```python
from build123d import *

# Parameters (mm, degrees)
F1_DEPTH   = 2
F2_DEPTH   = 7
F3_SIZE2   = 1.74999
F3_SIZE    = 0.99999
F3_2_SIZE2 = 1.74999
F3_2_SIZE  = 0.99999
F3_3_SIZE2 = 1.74999
F3_3_SIZE  = 0.99999
F3_4_SIZE2 = 1.74999
F3_4_SIZE  = 0.99999


# Not quite as in the source:
# - a fillet or chamfer is up to 0.001 mm smaller than in the source, because OpenCascade refuses the exact size


with BuildPart() as f1:
    # F0 (on Top) → F1 (new body)
    with BuildSketch(Plane.XY):
        with BuildLine():
            ThreePointArc((2.5497759502, -1.5807095255), (2.8852493697, -0.8217883394), (3, 0))
            ThreePointArc((3, 0), (2.6235481729, 1.4549896853), (1.5886700104, 2.544823687))
            ThreePointArc((1.5886700104, 2.544823687), (0.8262956308, 2.8839617769), (0, 3))
            ThreePointArc((0, 3), (-1.6310845521, 2.51784892), (-2.7378829853, 1.226375456))
            ThreePointArc((-2.7378829853, 1.226375456), (-2.9337389928, 0.6270370979), (-3, 0))
            ThreePointArc((-3, 0), (-2.488818496, -1.6750470125), (-1.1294783373, -2.7792586575))
            ThreePointArc((-1.1294783373, -2.7792586575), (-0.5754233343, -2.944297537), (0, -3))
            ThreePointArc((0, -3), (1.4590872872, -2.6212715022), (2.5497759502, -1.5807095255))
        make_face()
        with BuildLine():
            Line((0, -4.75), (0, -3))
            ThreePointArc((0, -3), (-0.5754233343, -2.944297537), (-1.1294783373, -2.7792586575))
            Line((-1.1294783373, -2.7792586575), (-2.0097266443, -4.3038934484))
            ThreePointArc((-2.0097266443, -4.3038934484), (-1.0293216504, -4.6371324048), (0, -4.75))
        make_face()
        with BuildLine():
            Line((4.75, 0), (3, 0))
            ThreePointArc((3, 0), (2.8852493697, -0.8217883394), (2.5497759502, -1.5807095255))
            Line((2.5497759502, -1.5807095255), (4.0657909798, -2.455981211))
            ThreePointArc((4.0657909798, -2.455981211), (4.5757516953, -1.2747534754), (4.75, 0))
        make_face()
        with BuildLine():
            ThreePointArc((-3, 0), (-2.9337389928, 0.6270370979), (-2.7378829853, 1.226375456))
            Line((-2.7378829853, 1.226375456), (-4.2584618162, 2.1042820533))
            ThreePointArc((-4.2584618162, 2.1042820533), (-4.625483414, 1.0804643384), (-4.75, 0))
            Line((-4.75, 0), (-3, 0))
        make_face()
        with BuildLine():
            ThreePointArc((0, 3), (0.8262956308, 2.8839617769), (1.5886700104, 2.544823687))
            Line((1.5886700104, 2.544823687), (2.4639985646, 4.0609372162))
            ThreePointArc((2.4639985646, 4.0609372162), (1.2792670212, 4.5744918722), (0, 4.75))
            Line((0, 4.75), (0, 3))
        make_face()
    extrude(amount=F1_DEPTH)

    # F0 (on Top) → F2 (join)
    with BuildSketch(Plane.XY):
        with BuildLine():
            Line((-2.0097266443, -4.3038934484), (-1.1294783373, -2.7792586575))
            ThreePointArc((-1.1294783373, -2.7792586575), (-2.488818496, -1.6750470125), (-3, 0))
            Line((-3, 0), (-4.75, 0))
            ThreePointArc((-4.75, 0), (-4.0067880877, -2.5511074497), (-2.0097266443, -4.3038934484))
        make_face()
        with BuildLine():
            Line((4.0657909798, -2.455981211), (2.5497759502, -1.5807095255))
            ThreePointArc((2.5497759502, -1.5807095255), (1.4590872872, -2.6212715022), (0, -3))
            Line((0, -3), (0, -4.75))
            ThreePointArc((0, -4.75), (2.334158226, -4.1369318795), (4.0657909798, -2.455981211))
        make_face()
        with BuildLine():
            ThreePointArc((1.5886700104, 2.544823687), (2.6235481729, 1.4549896853), (3, 0))
            Line((3, 0), (4.75, 0))
            ThreePointArc((4.75, 0), (4.1392326089, 2.3300758376), (2.4639985646, 4.0609372162))
            Line((2.4639985646, 4.0609372162), (1.5886700104, 2.544823687))
        make_face()
        with BuildLine():
            ThreePointArc((-2.7378829853, 1.226375456), (-1.6310845521, 2.51784892), (0, 3))
            Line((0, 3), (0, 4.75))
            ThreePointArc((0, 4.75), (-2.5067070278, 4.0347143488), (-4.2584618162, 2.1042820533))
            Line((-4.2584618162, 2.1042820533), (-2.7378829853, 1.226375456))
        make_face()
    extrude(amount=F2_DEPTH)

    # F3 (size 1 and 1.75 in the source; OpenCascade refuses exactly that, so slightly less here)
    f3_edges = [f1.edges().sort_by_distance(p)[0] for p in [
        (-2.488818, -1.675047, 7),
    ]]
    f3_side = f1.faces().sort_by_distance((-2.488818, -1.675047, 4.5))[0]
    chamfer(f3_edges, length=F3_SIZE, length2=F3_SIZE2, reference=f3_side)

    # F3#2 (size 1 and 1.75 in the source; OpenCascade refuses exactly that, so slightly less here)
    f3_2_edges = [f1.edges().sort_by_distance(p)[0] for p in [
        (-1.631085, 2.517849, 7),
    ]]
    f3_2_side = f1.faces().sort_by_distance((-1.631085, 2.517849, 4.5))[0]
    chamfer(f3_2_edges, length=F3_2_SIZE, length2=F3_2_SIZE2, reference=f3_2_side)

    # F3#3 (size 1 and 1.75 in the source; OpenCascade refuses exactly that, so slightly less here)
    f3_3_edges = [f1.edges().sort_by_distance(p)[0] for p in [
        (2.623548, 1.45499, 7),
    ]]
    f3_3_side = f1.faces().sort_by_distance((2.623548, 1.45499, 4.5))[0]
    chamfer(f3_3_edges, length=F3_3_SIZE, length2=F3_3_SIZE2, reference=f3_3_side)

    # F3#4 (size 1 and 1.75 in the source; OpenCascade refuses exactly that, so slightly less here)
    f3_4_edges = [f1.edges().sort_by_distance(p)[0] for p in [
        (1.459087, -2.621272, 7),
    ]]
    f3_4_side = f1.faces().sort_by_distance((1.459087, -2.621272, 4.5))[0]
    chamfer(f3_4_edges, length=F3_4_SIZE, length2=F3_4_SIZE2, reference=f3_4_side)


solid = f1.part
```
For this review, take the finished solid that the model builds, in its own axes (mm). A direction names the side the tool comes from. Round coordinates to 2 decimals unless told otherwise and drop trailing zeros. Write each loop counter-clockwise with the first axis right and the second up, starting at its lowest first coordinate (ties: lowest second). Pieces come first, ordered by that corner, then holes. Notation, with made-up numbers: (13, 28.25) -> (64, 28.25) arc R35 cw to (64, 65.25) -> close; hole circle Ø5 at (71.25, 43). An arc over 180 degrees is marked (long way). One line per question, with ' | ' between items. Start each with the question number.
1) Add section B-B (z = 1.5). Write out the cut boundary in (x, y).
2) For pin 1 Ø1 at (y, z) = (3, 3.5) entering from -X; pin 2 Ø1.9 at (x, z) = (-4, 4) entering from +Y; pin 3 Ø0.9 at (y, z) = (3.5, 4.5) entering from +X, all flat-tipped, find the tip position at first contact; note any pin that passes through.
3) Machinability: for faces 1 (the flat face through (0, -4, 4)), 2 (the flat face through (-3.51, 1.67, 4.46)), 3 (the flat face through (3.318, -2.024, 4.465)), 4 (the conical face through (3.205, 1.835, 6.396)), which of the approach directions +Z, -Z, +X, -X, +Y, -Y give a long, thin tool a straight path to every point of the face, cutting with its end or side? Answer none if there is none.
4) Add section C-C (z = 6.25). Write out the cut boundary in (x, y), and give its area (3 significant figures).
5) Mouldability with a two-part tool opening along Y and no side actions: class faces 5 (the flat face through (2.03, 3.31, 4.47)), 6 (the flat face through (4, 0, 4)), 7 (the flat face through (0, 0, 0)) as +Y half, -Y half, draft (parallel to the pull), parting line (faces both ways), or undercut.
6) Add section A-A (z = 3.5). Write out the cut boundary in (x, y), and give its area (3 significant figures).
7) Wall thickness on line 1 along Z through (x, y) = (0, 0.5); line 2 along X through (y, z) = (-1.75, 4.5); line 3 along X through (y, z) = (-2.75, 3.5): over which ranges is each line inside the solid? List them lowest first.
Reported:
1) outline: circle Ø9.5 at (0, 0)
2) pin 1: stops at x = -4.04 | pin 2: stops at y = 3.64 | pin 3: stops at x = 3.64
3) face 1: +Z, -Y | face 2: +Z, -X | face 3: +Z, +X | face 4: +Z
4) outline: (-4.75, 0) arc R4.75 ccw to (-2.01, -4.3) -> (-1.35, -3.16) arc R3.44 cw to (-3.44, 0) -> close; (-4.26, 2.1) -> (-3.12, 1.45) arc R3.44 cw to (0, 3.44) -> (0, 4.75) arc R4.75 ccw to start; (0, -4.75) arc R4.75 ccw to (4.07, -2.46) -> (2.93, -1.8) arc R3.44 cw to (0, -3.44) -> close; (1.81, 2.92) arc R3.44 cw to (3.44, 0) -> (4.75, 0) arc R4.75 ccw to (2.46, 4.06) -> close | area: 23.2 mm²
5) face 5: +Y half | face 6: undercut | face 7: draft
6) outline: (-4.75, 0) arc R4.75 ccw to (-2.01, -4.3) -> (-1.13, -2.78) arc R3 cw to (-3, 0) -> close; (-4.26, 2.1) -> (-2.74, 1.23) arc R3 cw to (0, 3) -> (0, 4.75) arc R4.75 ccw to start; (0, -4.75) arc R4.75 ccw to (4.07, -2.46) -> (2.55, -1.58) arc R3 cw to (0, -3) -> close; (1.59, 2.54) arc R3 cw to (3, 0) -> (4.75, 0) arc R4.75 ccw to (2.46, 4.06) -> close | area: 29.3 mm²
7) line 1: z = 0 to 2 | line 2: x = -4.42 to -2.44, 2.44 to 2.84 | line 3: x = -3.87 to -1.2, 1.2 to 3.87
